Autodesk Inventor part; units mm, degrees
ref_plane "YZ Plane" through (0, 0, 0) normal (1, 0, 0) x (0, 1, 0)
ref_plane "XZ Plane" through (0, 0, 0) normal (0, 1, 0) x (-1, 0, 0)
ref_plane "XY Plane" through (0, 0, 0) normal (0, 0, 1) x (1, 0, 0)
sketch "Sketch2" plane through (0, 0, 0) normal (0, 0, 1) x (1, 0, 0)
  line L0 (0, 0) -> (0, -10)
  line L1 (0, 0) -> (-27, 0)
  line L2 (-27, 0) -> (-27, 20)
  line L3 (-27, 20) -> (6, 20)
  line L4 (0, -10) -> (25, -10)
  line L5 (25, -10) -> (25, -4)
  line L6 (25, -4) -> (6, -4)
  line L7 (6, 20) -> (6, -4)
  dimension "d4" = 10
  dimension "d5" = 27
  dimension "d6" = 20
  dimension "d7" = 33
  dimension "d9" = 25
  dimension "d10" = 6
extrude "Extrusion6" add sketch "Sketch2" against normal blind 20
sketch "Sketch9" plane through (6, -4, 0) normal (1, 0, 0) x (0, 0, -1)
  line L0 (0, 4) -> (20, 4)
  line L1 (20, 24) -> (20, 0)
  line L2 (0, 4) -> (20, 24)
  arc A0 (4.8038, 13.25) -> (4.8038, 14.75) centre (10, 14) ccw
  line L3 (4.8038, 14.75) -> (0, 14.75)
  line L4 (4.8038, 13.25) -> (0, 13.25)
  line L5 (0, 13.25) -> (0, 14.75)
  line L6 (0, 0) -> (0, 24)
  dimension "d28" = 10.5
extrude "Extrusion7" cut sketch "Sketch9" against normal through all contours A0 L4 L5 L3 L2 | L2 A0
sketch "Sketch10" plane through (-27, 0, 0) normal (0, -1, 0) x (1, 0, 0)
  line L0 (33, 0) -> (0, 0)
  line L1 (0, 0) -> (6, 0)
  line L2 (6, 0) -> (6, -20)
  line L3 (6, -20) -> (0, -20)
  line L4 (0, -20) -> (0, 0)
  point P0 (27, 0)
  dimension "d33" = 6
  dimension "d34" = 20
extrude "Extrusion8" add sketch "Sketch10" along normal blind 10
sketch "Sketch11" plane through (-27, 20, -20) normal (-1, 0, 0) x (0, 0, 1)
  line L0 (20, -30) -> (0, -30)
  line L1 (20, -20) -> (20, -30)
  line L2 (0, -30) -> (20, -20)
  point P0 (10, -25)
hole "Hole1" at (-27, -5, -10) direction (1, 0, 0) diameter 5.5 end up to surface
sketch "Sketch13" plane through (0, -10, 0) normal (0, -1, 0) x (1, 0, 0)
  line L0 (0, -13) -> (25, -13)
  line L1 (0, -7) -> (25, -7)
  line L2 (0, -13) -> (0, -7)
  line L3 (0, 0) -> (0, -20)
  line L4 (25, -7) -> (25, -13)
  line L5 (0, 0) -> (25, 0)
  dimension "d69" = 25
extrude "Extrusion9" add sketch "Sketch13" along normal blind 1.5
sketch "Sketch14" plane through (0, -11.5, 0) normal (0, -1, 0) x (1, 0, 0)
  line L0 (0, -7) -> (25, -7)
  line L1 (25, -13) -> (0, -13)
  line L2 (0, -13) -> (25, -13)
  line L3 (25, 0) -> (25, -7)
  point P0 (0, 0)
  point P1 (15.5, -10)
  dimension "d70" = 9.5
hole "Hole2" at (15.5, -11.5, -10) direction (0, 1, 0) diameter 5.5 end through all counterbore diameter 10 counterbore depth 1.5
sketch "Sketch15" plane through (-27, 20, 0) normal (0, 1, 0) x (1, 0, 0)
  line L0 (33, 4.8038) -> (0, 4.8038)
  point P0 (27, 0)
  point P1 (16, 2.4019)
hole "Hole3" at (-11, 20, -2.4019) direction (0, -1, 0) diameter 4 end through all
sketch "Sketch16" plane through (0, 0, -20) normal (0, -1, 0) x (1, 0, 0)
  circle A0 centre (-11, 17.5981) radius 2
  line L0 (-7.4, 17.6276) -> (-9.1744, 14.4952)
  line L1 (-9.1744, 14.4952) -> (-12.7744, 14.4656)
  line L2 (-12.7744, 14.4656) -> (-14.6, 17.5685)
  line L3 (-14.6, 17.5685) -> (-12.8256, 20.701)
  line L4 (-12.8256, 20.701) -> (-9.2256, 20.7305)
  line L5 (-9.2256, 20.7305) -> (-7.4, 17.6276)
  point P0 (0, 20)
  point P1 (-11, 17.5981)
  dimension "d65" = 7.2
extrude "Extrusion10" cut sketch "Sketch16" against normal blind 3
fillet "Fillet2" radius 2 9 edges at (-24, -10, 0) (-24, -10, -20) (-27, 20, -10) (6, 20, -10) (-10.5, 20, -20) (-10.5, 20, 0) (25, -7, -20) (25, -4, -10) (25, -7, 0)
chamfer "Chamfer3" distance 5 angle 45 1 edges at (6, -4, -10)
properties part number "EixoXY - Canto"
Work out the finished part from the listing and answer in its coordinate system (mm). A direction names the side the tool comes from. Give positions to 0.01 mm unless a question says otherwise; leave off trailing zeros. Order: outer loops, then holes, each group sorted by start corner. A loop starts at its lowest first (then second) coordinate and runs counter-clockwise, first axis right, second up. Notation, with made-up numbers: (67, 11) - (100, 11) arc R31 ccw to (100, 49) - close; hole circle Ø8 at (81, 76). An arc over 180 degrees is marked (long way). Answer as CSV lines item,"result". Start each with the question number.
Q1. For faces 4 (the face through (-23.96, -9.43, -19.4)), 5 (the face through (-8.275, 1.479, -3.917)), 6 (the face through (-21, -2.7, -12.1)), determine the directions among +Z, -Z, +X, -X, +Y, -Y from which every point of the face is accessible in a straight line to the end or side of a thin tool.
Q2. Given pin 1 Ø4.5 at (x, z) = (-11, -2) entering from -Y; pin 2 Ø2 at (y, z) = (-4.5, -9) entering from +X; pin 3 Ø3 at (x, z) = (-24.5, -14) entering from -Y, each flat-ended and moving along its own axis, determine where each tip first touches the part or whether it passes through.
Q3. The part is cut by section C-C (y = -5). Write down the section's boundary in (x, z), then the cut area to 3 significant figures.
Q4. The part is cut by section A-A (z = -10). Give the number of separate pieces and of enclosed holes in the cut face, then the cut area to 3 significant figures.
Q5. Find the intervals of material crossed by L1, parallel to Y at x = -24.25, z = -10; L2, parallel to X at y = -7.9, z = -10; L3, parallel to X at y = -7.55, z = -10, in increasing order. Write a range as [from, to].
Q6. The part is cut by section B-B (y = 13.5). Write down the section's boundary in (x, z).
Q7. The part is cut by section D-D (x = -11). Write down the section's boundary in (y, z).
Q8. The mould has two halves that part along Z. Classify faces 1 (the face through (-23.96, -3.95, -7.46)), 2 (the face through (6, -11, -13)), 3 (the face through (6, 13.4, -14.3)): +Z half, -Z half, draft (parallel to the pull), parting line (faces both ways), or undercut.
Check result:
1,face 4,"-Z, -X, -Y"
1,face 5,"-Y"
1,face 6,"+Z, -Z, -Y"
2,pin 1,"stops at y = 3"
2,pin 2,"stops at x = 24.94"
2,pin 3,"stops at y = -10"
3,outline,"(-27, -20) - (-21, -20) - (-21, -12.75) - (-27, -12.75) - close; (-27, -7.25) - (-21, -7.25) - (-21, 0) - (-27, 0) - close; (0, -20) - (23, -20) arc R2 ccw to (24.73, -19) - (24.73, -1) arc R2 ccw to (23, 0) - (0, 0) - close; hole circle Ø5.5 at (15.5, -10)"
3,area,"557 mm²"
4,separate pieces,"4"
4,enclosed holes,"0"
4,area,"514 mm²"
5,L1,"y = [-10, -7.75], [-2.25, 4.75], [15.25, 20]"
5,L2,"x = [-27, -21], [0, 12.75], [18.25, 25]"
5,L3,"x = [0, 12.75], [18.25, 25]"
6,outline,"(-27, -20) - (6, -20) - (6, -13.91) - (-27, -13.91) - close; (-27, -6.09) - (6, -6.09) - (6, 0) - (-27, 0) - close; hole circle Ø4 at (-11, -2.4)"
7,outline,"(0, -20) - (18, -20) arc R2 ccw to (20, -18) - (20, -4.4) - (10.75, -4.4) - (10.75, -4.8) arc R5.25 cw (long way) to (9.25, -4.8) - (9.25, -4.4) - (3, -4.4) - (3, -5.52) - (0, -5.52) - close; (3, -0.4) - (9.25, -0.4) - (9.25, 0) - (3, 0) - close; (10.75, -0.4) - (19.2, -0.4) arc R2 ccw to (18, 0) - (10.75, 0) - close"
8,face 1,"undercut"
8,face 2,"-Z half"
8,face 3,"draft"
